```python
from build123d import *

# Parameters (mm, degrees)
SKETCH1_R                = 2
BOSS_EXTRUDE1_DEPTH      = 2.5
BOSS_EXTRUDE1_2_DEPTH    = 2.5
BOSS_EXTRUDE3_DEPTH      = 1
FILLET1_R                = 1
BOSS_EXTRUDE4_DEPTH      = 2
BOSS_EXTRUDE4_DEPTH_BACK = 1
SKETCH3_W                = 4.9
SKETCH3_H                = 5.030022666
SKETCH3_H_2              = 5.609354891
BOSS_EXTRUDE5_DEPTH      = 2
BOSS_EXTRUDE5_DEPTH_BACK = 7
SKETCH4_R                = 1
BOSS_EXTRUDE6_DEPTH      = 2
BOSS_EXTRUDE6_DEPTH_BACK = 7
SKETCH5_R                = 1
FILLET2_R                = 2
FILLET3_R                = 2
CUT_EXTRUDE1_DEPTH       = 0.5
FILLET4_R                = 2
FILLET6_R                = 2
SKETCH7_W                = 77.047719234
SKETCH7_H                = 13.468868212
CUT_EXTRUDE2_DEPTH       = 10
SKETCH8_R                = 1
BOSS_EXTRUDE7_DEPTH      = 4
BOSS_EXTRUDE7_2_DEPTH    = 4
BOSS_EXTRUDE8_DEPTH      = 1
SKETCH10_W               = 70.230539596
SKETCH10_H               = 4.186533739
CUT_EXTRUDE4_DEPTH       = 1


# Some blends are built 0.0001 mm under size
with BuildPart() as part:
    # Sketch1 → Boss-Extrude1 (new body)
    with BuildSketch(Plane(origin=(0, 0, 0), x_dir=(1, 0, 0), z_dir=(0, 1, 0))):
        with Locations(Location((67.22, 0, 0), (0, 0, 270))):
            Circle(SKETCH1_R)
    extrude(amount=BOSS_EXTRUDE1_DEPTH)



with BuildPart() as body_2:
    # Sketch1 → Boss-Extrude1 2 (new body)
    with BuildSketch(Plane(origin=(0, 0, 0), x_dir=(1, 0, 0), z_dir=(0, 1, 0))):
        with Locations(Location((0, 0, 0), (0, 0, 270))):
            Circle(SKETCH1_R)
    extrude(amount=BOSS_EXTRUDE1_2_DEPTH)


with BuildPart() as part_1:
    add(part.part)

    add(body_2.part)  # Boss-Extrude3 merges body 2
    # Sketch2 → Boss-Extrude3 (add)
    with BuildSketch(Plane(origin=(0, 2.5, 0), x_dir=(1, 0, 0), z_dir=(0, 1, 0))):
        Polygon((0, 3.373067478), (0, 8), (67.22031246, 8), (67.22031246, 3.373067478), (69.745167769, 3.373067478), (69.745167769, -3.373067478), (-2.485371827, -3.373067478), (-2.485371827, 3.373067478), align=None)
    extrude(amount=BOSS_EXTRUDE3_DEPTH)

    # Fillet1
    fillet1_edges = [part_1.edges().sort_by_distance(p)[0] for p in [
        (67.22031246, 3, -3.373067478),
        (0, 3, -3.373067478),
        (-2.485371827, 3, -3.373067478),
        (-2.485371827, 3, 3.373067478),
        (69.745167769, 3, 3.373067478),
        (69.745167769, 3, -3.373067478),
    ]]
    fillet(fillet1_edges, radius=FILLET1_R)

    # Sketch3 → Boss-Extrude4 (add, two sides: drawn at the far end of the back side and taken through both)
    with BuildSketch(Plane(origin=(0, 3.5, 0), x_dir=(1, 0, 0), z_dir=(0, 1, 0)).offset(-BOSS_EXTRUDE4_DEPTH_BACK)):
        with Locations((7.93, 9.710321272)):
            Rectangle(SKETCH3_W, SKETCH3_H)
        with Locations((56.17, 9.42065516)):
            Rectangle(SKETCH3_W, SKETCH3_H_2)
    extrude(amount=BOSS_EXTRUDE4_DEPTH + BOSS_EXTRUDE4_DEPTH_BACK)

    # Sketch4 → Boss-Extrude5 (add, two sides: drawn at the far end of the back side and taken through both)
    with BuildSketch(Plane.ZY.offset(-5.48).offset(-BOSS_EXTRUDE5_DEPTH_BACK)):
        with Locations((-12.225332605, 5.316497078)):
            Circle(SKETCH4_R)
    extrude(amount=BOSS_EXTRUDE5_DEPTH + BOSS_EXTRUDE5_DEPTH_BACK)

    # Sketch5 → Boss-Extrude6 (add, two sides: drawn at the far end of the back side and taken through both)
    with BuildSketch(Plane.ZY.offset(-53.72).offset(-BOSS_EXTRUDE6_DEPTH_BACK)):
        with Locations((-12.225332605, 5.316497078)):
            Circle(SKETCH5_R)
    extrude(amount=BOSS_EXTRUDE6_DEPTH + BOSS_EXTRUDE6_DEPTH_BACK)

    # Fillet2
    fillet2_edges = [part_1.edges().sort_by_distance(p)[0] for p in [
        (7.93, 5.5, -7.195309939),
        (56.17, 5.5, -6.615977714),
    ]]
    fillet(fillet2_edges, radius=FILLET2_R - 0.0001)  # a hair under: the kernel refuses the full size

    # Fillet3
    # the kernel refuses this fillet: 2 mm, written as the material it takes off along each edge
    with BuildSketch(Plane(origin=(48.741090307, 2.5, -12.225332605), x_dir=(0, 0, 1), z_dir=(1, 0, 0))) as fillet3_piece_1:
        with BuildLine():
            CenterArc((1.991563877, -2), FILLET3_R, 90, 84.735624625)
            Line((0, -1.816497078), (-0.039831278, -1.81282702))
            ThreePointArc((-0.039831278, -1.81282702), (-0.04, -0.908248539), (-0.04, 0))
            Line((-0.04, 0), (0, 0.04))
            Line((0, 0.04), (1.991563877, 0.04))
            Line((1.991563877, 0.04), (1.991563877, 0))
        make_face()
    extrude(amount=14.857819387, mode=Mode.SUBTRACT)

    # Sketch6 → Cut-Extrude1 (cut)
    with BuildSketch(Plane(origin=(0, 3.5, 0), x_dir=(1, 0, 0), z_dir=(0, 1, 0))):
        with BuildLine():
            Line((59.62, 5.615977714), (52.72, 5.615977714))
            Line((52.72, 5.615977714), (52.72, 7))
            Line((52.72, 7), (11.38, 7))
            Line((11.38, 7), (11.38, 6.195309939))
            Line((11.38, 6.195309939), (4.48, 6.195309939))
            Line((4.48, 6.195309939), (4.48, 7))
            Line((4.48, 7), (1, 7))
            Line((1, 7), (1, 4.373067478))
            ThreePointArc((1, 4.373067478), (0.414213562, 2.958853916), (-1, 2.373067478))
            Line((-1, 2.373067478), (-1.485371827, 2.373067478))
            Line((-1.485371827, 2.373067478), (-1.485371827, -2.373067478))
            Line((-1.485371827, -2.373067478), (68.745167769, -2.373067478))
            Line((68.745167769, -2.373067478), (68.745167769, 2.373067478))
            Line((68.745167769, 2.373067478), (68.22031246, 2.373067478))
            ThreePointArc((68.22031246, 2.373067478), (66.806098898, 2.958853916), (66.22031246, 4.373067478))
            Line((66.22031246, 4.373067478), (66.22031246, 7))
            Line((66.22031246, 7), (59.62, 7))
            Line((59.62, 7), (59.62, 5.615977714))
        make_face()
    extrude(amount=-CUT_EXTRUDE1_DEPTH, mode=Mode.SUBTRACT)

    # Fillet4
    # the kernel refuses this fillet: 2 mm, written as the material it takes off along each edge
    with BuildSketch(Plane(origin=(15.358909693, 2.5, -12.225332605), x_dir=(0, 0, 1), z_dir=(-1, 0, 0))) as fillet4_piece_1:
        with BuildLine():
            CenterArc((1.991563877, 2), FILLET4_R, 185.264375375, 84.735624625)
            Line((0, 1.816497078), (-0.039831278, 1.81282702))
            ThreePointArc((-0.039831278, 1.81282702), (-0.04, 0.908248539), (-0.04, 0))
            Line((-0.04, 0), (0, -0.04))
            Line((0, -0.04), (1.991563877, -0.04))
            Line((1.991563877, -0.04), (1.991563877, 0))
        make_face()
    extrude(amount=14.857819387, mode=Mode.SUBTRACT)

    # Fillet6
    fillet6_edges = [part_1.edges().sort_by_distance(p)[0] for p in [
        (67.22031246, 3, -8),
        (0, 3, -8),
    ]]
    fillet(fillet6_edges, radius=FILLET6_R)

    # Sketch7 → Cut-Extrude2 (cut)
    with BuildSketch(Plane.XZ.offset(-2.5)):
        with Locations((32.181632572, 2.423814337)):
            Rectangle(SKETCH7_W, SKETCH7_H)
    extrude(amount=CUT_EXTRUDE2_DEPTH, mode=Mode.SUBTRACT)



with BuildPart() as body_2_2:
    # Sketch8 → Boss-Extrude7 (new body)
    with BuildSketch(Plane(origin=(0, 2.5, 0), x_dir=(-1, 0, 0), z_dir=(0, -1, 0))):
        with Locations(Location((3.870102029, 0, 0), (0, 0, 90))):
            Circle(SKETCH8_R)
    extrude(amount=BOSS_EXTRUDE7_DEPTH)


with BuildPart() as body_3:
    # Sketch8 → Boss-Extrude7 2 (new body)
    with BuildSketch(Plane(origin=(0, 2.5, 0), x_dir=(-1, 0, 0), z_dir=(0, -1, 0))):
        with Locations(Location((-71.129897971, 0, 0), (0, 0, 90))):
            Circle(SKETCH8_R)
    extrude(amount=BOSS_EXTRUDE7_2_DEPTH)


with BuildPart() as part_2:
    add(part_1.part)

    add(body_2_2.part)  # Boss-Extrude8 merges body 2 2

    add(body_3.part)  # Boss-Extrude8 merges body 3
    # Sketch9 → Boss-Extrude8 (add)
    with BuildSketch(Plane.XZ.offset(-2.5)):
        with BuildLine():
            Line((-3.870102029, 2), (71.129897971, 2))
            ThreePointArc((71.129897971, 2), (73.129897971, 0), (71.129897971, -2))
            Line((71.129897971, -2), (-3.870102029, -2))
            ThreePointArc((-3.870102029, -2), (-5.870102029, 0), (-3.870102029, 2))
        make_face()
    extrude(amount=-BOSS_EXTRUDE8_DEPTH)

    # Sketch10 → Cut-Extrude4 (cut)
    with BuildSketch(Plane(origin=(0, 3, 0), x_dir=(1, 0, 0), z_dir=(0, 1, 0))):
        with Locations((33.629897971, -0.09326687)):
            Rectangle(SKETCH10_W, SKETCH10_H)
    extrude(amount=CUT_EXTRUDE4_DEPTH, mode=Mode.SUBTRACT)


solid = part_2.part
```
Source: CAD feature listing. Evaluate the final solid. Frame: model axes, mm. A direction names the side the tool comes from. Coordinates: 2 decimals unless noted, no trailing zeros. Order: outer loops, then holes, each group sorted by start corner. A loop starts at its lowest first (then second) coordinate and runs counter-clockwise, first axis right, second up. Notation, with made-up numbers: (2.5, -6) - (32.5, -6) arc R20 ccw to (32.5, 5) - close; hole circle Ø7 at (-21.5, -39). An arc over 180 degrees is marked (long way). One line per item, written item: value.
1) Contact query for flat-ended pins moving along their axis: pin 1 (0.5 mm diameter, centred on x = 23.5, y = 3, fed in from -Z); pin 2 (9 mm diameter, centred on x = 37, z = 0, fed in from +Y); pin 3 (3 mm diameter, centred on y = 2.5, z = -7, fed in from -X). Output: stop coordinate, or through.
Computed values:
pin 1: stops at z = -8
pin 2: stops at y = 3.5
pin 3: stops at x = 0
2) Cut plane B-B on x = 36. Output: boundary loops of the cut face in (y, z), plus the area to 3 significant figures.
Computed values:
outline: (2.5, -8) - (3.5, -8) - (3.5, -7) - (3, -7) - (3, 2.37) - (3.5, 2.37) - (3.5, 3.37) - (2.5, 3.37) - close
area: 6.69 mm^2
3) Cut plane A-A on z = 0. Output: boundary loops of the cut face in (x, y).
Computed values:
outline: (-5.87, 2.5) - (-4.87, 2.5) - (-4.87, -1.5) - (-2.87, -1.5) - (-2.87, 2.5) - (70.13, 2.5) - (70.13, -1.5) - (72.13, -1.5) - (72.13, 2.5) - (73.13, 2.5) - (73.13, 3.5) - (68.75, 3.5) - (68.75, 3) - (-1.49, 3) - (-1.49, 3.5) - (-5.87, 3.5) - close
4) Ray query, line 1 (Y direction, x = 66.5, z = 1); line 2 (X direction, y = 4.5, z = -12.5); line 3 (X direction, y = 3, z = -9.5). Return the intervals inside material, ascending. Write a range as [from, to].
Computed values:
line 1: y = [2.5, 3]
line 2: x = [3.48, 12.48], [51.72, 60.72]
line 3: x = [5.48, 10.38], [53.72, 58.62]
5) Mould query, pull axis X, two halves, no side actions, for faces 1 (the face through (51.72, 5, -12)), 2 (the face through (66.65, 3.01, -7.4)), 3 (the face through (34, 2.5, -2)), 4 (the face through (56, 5.5, -10)). Classes: released by +X, released by -X, zero draft, split by the parting line, or undercut.
Computed values:
face 1: undercut
face 2: released by +X
face 3: undercut
face 4: zero draft
6) Cut plane C-C on y = 0.25. Output: boundary loops of the cut face in (x, z).
Computed values:
outline: circle Ø2 at (-3.87, 0); circle Ø2 at (71.13, 0)
7) Reachability of faces 5 (the face through (0.43, 3.254, -2.974)), 6 (the face through (8, 5.5, -10)), 7 (the face through (7.964, 4.899, -7.766)) from +Z, -Z, +X, -X, +Y, -Y: full face, straight path, thin tool, end or side. Return the list, or none.
Computed values:
face 5: +Y
face 6: +Z, +X, -X, +Y
face 7: +Z, -X, +Y
